Design review of the part built by this model. Coordinates are the model's own, in mm. Face numbers are marked on the shaded views. A direction names the side the tool comes from. Give positions to 0.01 mm unless a question says otherwise; leave off trailing zeros. Order: outer loops, then holes, each group sorted by start corner. A loop starts at its lowest first (then second) coordinate and runs counter-clockwise, first axis right, second up. Notation, with made-up numbers: (78, 67) -> (117, 67) arc R26 cw to (117, 89) -> close; hole circle Ø10 at (26, -17.75). An arc over 180 degrees is marked (long way). Answer in a Markdown table with one row per item. Add a question column.
```python
from build123d import *

# Parameters (mm, degrees)
SKETCH1_W               = 137.16
SKETCH1_H               = 160.02
BOSS_EXTRUDE1_DEPTH     = 71.12
CUT_EXTRUDE1_DEPTH      = 174.99
CUT_EXTRUDE1_DEPTH_BACK = 174.99
SKETCH2_W               = 23.227349815
SKETCH2_H               = 32.529214904
FILLET1_R               = 2.54
FILLET2_R               = 2.54
SKETCH3_R               = 3.302
CUT_EXTRUDE2_DEPTH      = 7.62


with BuildPart() as part:
    # Sketch1 → Boss-Extrude1 (new body)
    with BuildSketch(Plane(origin=(0, 0, 0), x_dir=(1, 0, 0), z_dir=(0, 1, 0))):
        Rectangle(SKETCH1_W, SKETCH1_H)
    extrude(amount=-BOSS_EXTRUDE1_DEPTH)

    # Sketch2 → Cut-Extrude1 (cut, two sides: drawn at the far end of the back side and taken through both)
    with BuildSketch(Plane(origin=(68.58, 0, 0), x_dir=(0, 0, -1), z_dir=(1, 0, 0)).offset(-CUT_EXTRUDE1_DEPTH_BACK)):
        with Locations((-68.396325093, -16.264607452)):
            Rectangle(SKETCH2_W, SKETCH2_H)
        with Locations((68.396325093, -16.264607452)):
            Rectangle(SKETCH2_W, SKETCH2_H)
    extrude(amount=CUT_EXTRUDE1_DEPTH + CUT_EXTRUDE1_DEPTH_BACK, mode=Mode.SUBTRACT)

    # Fillet1
    fillet1_edges = [part.edges().sort_by_distance(p)[0] for p in [
        (68.58, 0, 0),
        (-68.58, 0, 0),
        (0, -71.12, 80.01),
        (68.58, -32.529214904, 68.396325092),
        (68.58, -16.264607452, 56.782650185),
        (0, -32.529214904, 80.01),
        (-68.58, -16.264607452, 56.782650185),
        (0, 0, 56.782650185),
        (-68.58, -32.529214904, 68.396325092),
        (0, -32.529214904, 56.782650185),
        (68.58, -32.529214904, -68.396325092),
        (68.58, -16.264607452, -56.782650185),
        (-68.58, -16.264607452, -56.782650185),
        (0, -32.529214904, -56.782650185),
        (0, 0, -56.782650185),
        (-68.58, -32.529214904, -68.396325092),
        (0, -32.529214904, -80.01),
        (68.58, -71.12, 0),
        (68.58, -51.824607452, 80.01),
        (-68.58, -51.824607452, 80.01),
        (68.58, -51.824607452, -80.01),
    ]]
    fillet(fillet1_edges, radius=FILLET1_R)

    # Fillet2
    # the kernel refuses this fillet: 2.54 mm, written as the material it takes off along each edge
    with BuildSketch(Plane(origin=(-66.04, -68.58, 77.47), x_dir=(-1, 0, 0), z_dir=(0, -1, 0))) as fillet2_piece_1_section:
        Polygon((0, 0), (FILLET2_R, 0), (FILLET2_R, -FILLET2_R), (0, -FILLET2_R), align=None)
    fillet2_piece_1 = extrude(amount=FILLET2_R, mode=Mode.PRIVATE)
    fillet2_piece_1 = fillet2_piece_1 - Plane(origin=(-66.04, -68.58, 77.47), x_dir=(0.7071067811865475, 0, -0.7071067811865476), z_dir=(0, -1, 0)) * Sphere(FILLET2_R, mode=Mode.PRIVATE)
    add(fillet2_piece_1, mode=Mode.SUBTRACT)
    with BuildSketch(Plane(origin=(-66.04, -35.069214904, -77.47), x_dir=(-1, 0, 0), z_dir=(0, 0, -1))) as fillet2_piece_2_section:
        Polygon((0, 0), (FILLET2_R, 0), (FILLET2_R, FILLET2_R), (0, FILLET2_R), align=None)
    fillet2_piece_2 = extrude(amount=FILLET2_R, mode=Mode.PRIVATE)
    fillet2_piece_2 = fillet2_piece_2 - Plane(origin=(-66.04, -35.069214904, -77.47), x_dir=(0.7071067811865475, -0.7071067811865475, 0), z_dir=(0, 0, -1)) * Sphere(FILLET2_R, mode=Mode.PRIVATE)
    add(fillet2_piece_2, mode=Mode.SUBTRACT)
    with BuildSketch(Plane(origin=(-68.58, -71.12, 77.47), x_dir=(1, 0, 0), z_dir=(0, 0, -1))) as fillet2_piece_3:
        with BuildLine():
            CenterArc((FILLET2_R, -FILLET2_R), FILLET2_R, 90, 90)
            Line((0, -FILLET2_R), (0, 0))
            Line((0, 0), (FILLET2_R, 0))
        make_face()
    extrude(amount=163.83, mode=Mode.SUBTRACT)
    with BuildSketch(Plane(origin=(-68.58, -35.069214904, -80.01), x_dir=(1, 0, 0), z_dir=(0, -1, 0))) as fillet2_piece_4:
        with BuildLine():
            CenterArc((FILLET2_R, FILLET2_R), FILLET2_R, 180, 90)
            Line((0, FILLET2_R), (0, 0))
            Line((0, 0), (FILLET2_R, 0))
        make_face()
    extrude(amount=42.400785096, mode=Mode.SUBTRACT)

    # Sketch3 → Cut-Extrude2 (cut)
    with BuildSketch(Plane.XZ.offset(71.12)):
        with Locations(Location((-22.2504, -57.4675, 0), (0, 0, 270))):
            Circle(SKETCH3_R)
        with Locations(Location((-22.2504, 57.4675, 0), (0, 0, 270))):
            Circle(SKETCH3_R)
        with Locations(Location((22.2504, 57.4675, 0), (0, 0, 270))):
            Circle(SKETCH3_R)
        with Locations(Location((22.2504, -57.4675, 0), (0, 0, 270))):
            Circle(SKETCH3_R)
    extrude(amount=-CUT_EXTRUDE2_DEPTH, mode=Mode.SUBTRACT)


solid = part.part
```
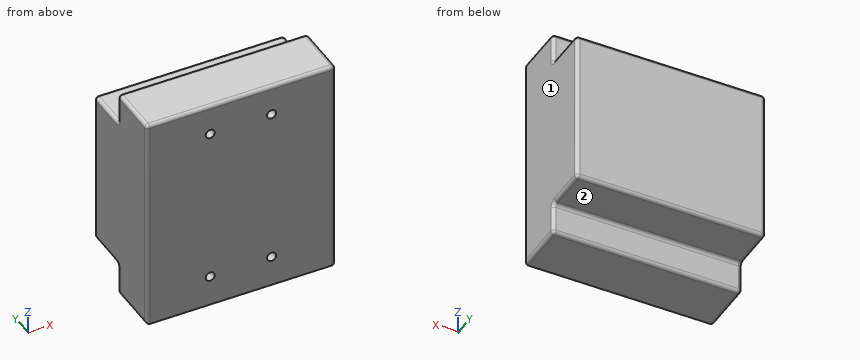
1) Clearance check with flat-ended pins moving along their axes: P1, Ø3.5, axis at x = -21.5, z = 57, coming from the -Y side; P2, Ø8, axis at x = 34, y = -24.5, coming from the +Z side; P3, Ø5.5, axis at x = -22.25, z = 57.47, coming from the +Y side. State where each tip first meets the part, or that it passes through.
2) Machinability: for the marked faces 1 and 2, which of the approach directions +Z, -Z, +X, -X, +Y, -Y give a long, thin tool a straight path to every point of the face, cutting with its end or side? Answer none if there is none.
3) Add section A-A, the plane y = -24. Write out the cut boundary in (x, z), and give its area (3 significant figures).
4) For L1, parallel to Z at x = 35.5, y = -21; L2, parallel to Y at x = 59, z = -63.5; L3, parallel to Z at x = -29.5, y = -31, list the stretches that pass through material, from the lowest coordinate up.
5) Add section B-B, the plane x = 29. Write out the cut boundary in (y, z).
Verdict:
| question | item | result |
|---|---|---|
| 1 | P1 | stops at y = -63.5 |
| 1 | P2 | stops at z = 56.78 |
| 1 | P3 | stops at y = -0.05 |
| 2 | face 1 | +Z, -Z, +X, +Y, -Y |
| 2 | face 2 | -Z, +X, -X, +Y |
| 3 | outline | (-68.58, -54.24) arc R2.54 ccw to (-66.04, -56.78) -> (66.04, -56.78) arc R2.54 ccw to (68.58, -54.24) -> (68.58, 54.24) arc R2.54 ccw to (66.04, 56.78) -> (-66.04, 56.78) arc R2.54 ccw to (-68.58, 54.24) -> close |
| 3 | area | 15,600 mm2 |
| 4 | L1 | z = -56.78 to 56.78 |
| 4 | L2 | y = -71.12 to -32.53 |
| 4 | L3 | z = -56.99 to 56.99 |
| 5 | outline | (-71.12, -80.01) -> (-35.07, -80.01) arc R2.54 ccw to (-32.53, -77.47) -> (-32.53, -59.32) arc R2.54 cw to (-29.99, -56.78) -> (-2.54, -56.78) arc R2.54 ccw to (0, -54.24) -> (0, 54.24) arc R2.54 ccw to (-2.54, 56.78) -> (-29.99, 56.78) arc R2.54 cw to (-32.53, 59.32) -> (-32.53, 77.47) arc R2.54 ccw to (-35.07, 80.01) -> (-68.58, 80.01) arc R2.54 ccw to (-71.12, 77.47) -> close |
